```python
from build123d import *

# Parameters (mm, degrees)
SKETCH1_W           = 120
SKETCH1_H           = 120
BOSS_EXTRUDE1_DEPTH = 6


with BuildPart() as part:
    # Sketch1 → Boss-Extrude1 (new body)
    with BuildSketch(Plane(origin=(0, 0, 0), x_dir=(0, 1, 0), z_dir=(0, 0, 1))):
        Rectangle(SKETCH1_W, SKETCH1_H)
    extrude(amount=BOSS_EXTRUDE1_DEPTH)

    # Sketch7 → CBORE for M3 SBHCS1 (revolve, cut)
    with BuildSketch(Plane(origin=(-55, 55, 6), x_dir=(0, -1, 0), z_dir=(1, 0, 0))):
        Polygon((0, 0), (0, 6), (1.25, 6), (1.25, 3), (3.25, 3), (3.25, 0.125), (3.375, 0), align=None)
    cbore_for_m3_sbhcs1 = revolve(axis=Axis((-55, 55, 12.35), (0, 0, -1)), mode=Mode.SUBTRACT)

    # Mirror2: CBORE for M3 SBHCS1 across plane
    add(cbore_for_m3_sbhcs1.mirror(Plane(origin=(0, 0, 0), x_dir=(0, 0, 1), z_dir=(1, 0, 0))), mode=Mode.SUBTRACT)

    # Mirror2 at the second plane: CBORE for M3 SBHCS1 across plane
    add(cbore_for_m3_sbhcs1.mirror(Plane.ZX), mode=Mode.SUBTRACT)

    # Mirror2 at the second plane copy 1 sketc → Mirror2 at the second plane copy 1 (revolve, cut)
    with BuildSketch(Plane(origin=(55, -55, 6), x_dir=(0, 1, 0), z_dir=(-1, 0, 0))):
        Polygon((0, 0), (0, 6), (1.25, 6), (1.25, 3), (3.25, 3), (3.25, 0.125), (3.375, 0), align=None)
    revolve(axis=Axis((55, -55, 12.35), (0, 0, -1)), mode=Mode.SUBTRACT)


solid = part.part
```
The listing builds one solid part. Answer for the finished solid, in the listing's coordinates (mm). A direction names the side the tool comes from. Round coordinates to 2 decimals unless told otherwise and drop trailing zeros. Use CSV: the item, a comma, the result in double quotes. Start each with the question number.
(1) The mould has two halves that part along X. Classify faces 1 (the face through (53.022, 57.579, 4.458)), 2 (the face through (60, -1, 3)), 3 (the face through (-55.05, -56.4, 3)), 4 (the face through (-60, -1, 3)): released by +X, released by -X, zero draft, split by the parting line, or undercut.
(2) Consider L1, parallel to X at y = -55, z = 2.3; L2, parallel to Y at x = -55, z = 5. Determine where each line is inside the solid, lowest interval first. Write a range as from..to.
(3) This flat-tipped pin is pushed along its axis until it touches: pin 1 (3 mm diameter, centred on x = -55, y = -56.5, fed in from +Z). Where does it stop, or does it pass through?
(4) Which of the six approach directions +Z, -Z, +X, -X, +Y, -Y give full straight-line access (tool end or side, diameter ignored) to faces 5 (the face through (-1, -1, 6)), 6 (the face through (53.022, -57.579, 4.458))?
A:
1,face 1,"undercut"
1,face 2,"released by +X"
1,face 3,"undercut"
1,face 4,"released by -X"
2,L1,"x = -60..-56.25, -53.75..53.75, 56.25..60"
2,L2,"y = -60..-58.25, -51.75..51.75, 58.25..60"
3,pin 1,"stops at z = 3"
4,face 5,"+Z, +X, -X, +Y, -Y"
4,face 6,"+Z"
